Can you work these out from the model? Positions are in its coordinate system, mm. Face numbers are marked on the shaded views. A direction names the side the tool comes from. Coordinates: 2 decimals unless noted, no trailing zeros. Order: outer loops, then holes, each group sorted by start corner. A loop starts at its lowest first (then second) coordinate and runs counter-clockwise, first axis right, second up. Notation, with made-up numbers: (2, 73.5) -> (24, 73.5) arc R25 cw to (24, 106.5) -> close; hole circle Ø1 at (33.25, -9.75). An arc over 180 degrees is marked (long way). Answer in a Markdown table with one row per item.
```python
from build123d import *

# Parameters (mm, degrees)
SKETCH1_R           = 15
BOSS_EXTRUDE1_DEPTH = 10
SKETCH2_W           = 7
SKETCH2_H           = 15
BOSS_EXTRUDE2_DEPTH = 10
CIRPATTERN1_COUNT   = 6


with BuildPart() as part:
    # Sketch1 → Boss-Extrude1 (new body)
    with BuildSketch(Plane.XY):
        Circle(SKETCH1_R)
    extrude(amount=BOSS_EXTRUDE1_DEPTH)

    # Sketch2 → Boss-Extrude2 (add)
    with BuildSketch(Plane.XY.offset(10)):
        with Locations((0, 15)):
            Rectangle(SKETCH2_W, SKETCH2_H)
    boss_extrude2 = extrude(amount=-BOSS_EXTRUDE2_DEPTH)

    # CirPattern1: Boss-Extrude2 ×6 about axis
    cirpattern1_axis = Axis((0, 0, 0), (0, 0, 1))
    for i in range(1, CIRPATTERN1_COUNT):
        add(boss_extrude2.rotate(cirpattern1_axis, i * 360 / CIRPATTERN1_COUNT))


solid = part.part
```
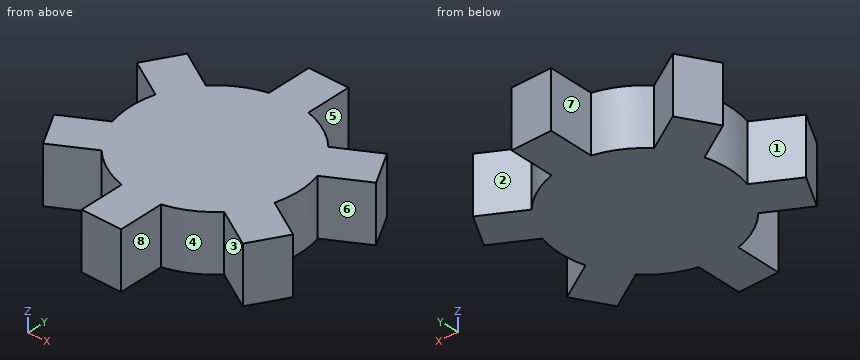
(1) Suppose I cut it at B-B (x = 18.5). Please give me the cut outline in (y, z), and give its area (3 significant figures).
Response values:
| item | result |
|---|---|
| outline | (-12.96, 0) -> (-6.64, 0) -> (-6.64, 10) -> (-12.96, 10) -> close; (6.64, 0) -> (12.96, 0) -> (12.96, 10) -> (6.64, 10) -> close |
| area | 126 mm2 |
(2) Suppose I cut it at C-C (z = 3.25). Please give me the cut outline in (x, y).
Response values:
| item | result |
|---|---|
| outline | (-21.24, -8.22) -> (-17.74, -14.28) -> (-10.88, -10.32) arc R15 ccw to (-3.5, -14.59) -> (-3.5, -22.5) -> (3.5, -22.5) -> (3.5, -14.59) arc R15 ccw to (10.88, -10.32) -> (17.74, -14.28) -> (21.24, -8.22) -> (14.38, -4.26) arc R15 ccw to (14.38, 4.26) -> (21.24, 8.22) -> (17.74, 14.28) -> (10.88, 10.32) arc R15 ccw to (3.5, 14.59) -> (3.5, 22.5) -> (-3.5, 22.5) -> (-3.5, 14.59) arc R15 ccw to (-10.88, 10.32) -> (-17.74, 14.28) -> (-21.24, 8.22) -> (-14.38, 4.26) arc R15 ccw to (-14.38, -4.26) -> close |
(3) Suppose I cut it at D-D (y = -12). Please give me the cut outline in (x, z).
Response values:
| item | result |
|---|---|
| outline | (-19.05, 0) -> (-13.78, 0) -> (-13.78, 10) -> (-19.05, 10) -> close; (-9, 0) -> (9, 0) -> (9, 10) -> (-9, 10) -> close; (13.78, 0) -> (19.05, 0) -> (19.05, 10) -> (13.78, 10) -> close |
(4) Suppose I cut it at A-A (y = 11). Please give me the cut outline in (x, z), and give its area (3 significant figures).
Response values:
| item | result |
|---|---|
| outline | (-19.63, 0) -> (-12.05, 0) -> (-12.05, 10) -> (-19.63, 10) -> close; (-10.2, 0) -> (10.2, 0) -> (10.2, 10) -> (-10.2, 10) -> close; (12.05, 0) -> (19.63, 0) -> (19.63, 10) -> (12.05, 10) -> close |
| area | 356 mm2 |
(5) On a 3-axis mill with a long thin cutter (end or side, diameter ignored), from which of +Z, -Z, +X, -X, +Y, -Y can I reach the whole of each face in a straight line? I mean the marked faces 4, 5, 6, 7 and 8. Say none if no direction works.
Response values:
| item | result |
|---|---|
| face 4 | +Z, -Z, -Y |
| face 5 | +Z, -Z, +X, +Y |
| face 6 | +Z, -Z, +X |
| face 7 | +Z, -Z, -X, +Y |
| face 8 | +Z, -Z, +X, -Y |
(6) I need wall thicknesses on line 1 (X direction, y = 16.5, z = 3); line 2 (Y direction, x = -17, z = 1); line 3 (Y direction, x = 19.5, z = 7) (3 decimals). Which ranges of each line are inside material? Lowest first, please. Write a range as [from, to].
Response values:
| item | result |
|---|---|
| line 1 | [-3.5, 3.5] |
| line 2 | [-13.86, -5.77], [5.77, 13.86] |
| line 3 | [-11.225, -7.217], [7.217, 11.225] |
(7) Will these pins go through, and if not, where does the flat tip stop? pin 1 Ø4 at (y, z) = (-17, 5.5) entering from +X; pin 2 Ø2 at (x, z) = (15.5, 3) entering from +Y.
Response values:
| item | result |
|---|---|
| pin 1 | x = 3.5 |
| pin 2 | y = 13.57 |
(8) We'd pull the mould along Y, two halves only. Please class the marked faces 1, 2 and 3: +Y half, -Y half, draft (parallel to the pull), parting line (faces both ways), or undercut.
Response values:
| item | result |
|---|---|
| face 1 | undercut |
| face 2 | +Y half |
| face 3 | -Y half |
